Can you work these out from the model? Positions are in its coordinate system, mm. Face numbers are marked on the shaded views. Give positions to 0.01 mm unless a question says otherwise; leave off trailing zeros. Return JSON: item names as keys, results as strings. Group by question number.
Q1. Suppose I cut it at A-A, the plane y = -104.5. Count the separate pieces of the cut face and the enclosed holes in it, and give its area (3 significant figures).
Q2. I need wall thicknesses on line 1 along Z through (x, y) = (0, -60); line 2 along Y through (x, z) = (70, 57). Which ranges of each line are inside material? Lowest first, please. Write a range as [from, to].
Q3. Will these pins go through, and if not, where does the flat tip stop? pin 1 (4 mm diameter, centred on y = -73, z = -92, fed in from -X); pin 2 (5.5 mm diameter, centred on y = -88, z = 89, fed in from -X); pin 3 (1.7 mm diameter, centred on x = 0, y = -80.5, fed in from -Z); pin 4 (4 mm diameter, centred on y = -79.5, z = -0.5, fed in from +X).
Q4. Thinking about a two-plate mould opening in Z: for the marked faces 1, 2 and 3, which applies, pulls with the +Z half, pulls with the -Z half, needs draft (parallel to the pull), parting line crosses it, or undercut?
```python
from build123d import *

# Parameters (mm, degrees)
SKETCH1_R           = 94.2975
SKETCH1_R_2         = 89.662
BOSS_EXTRUDE1_DEPTH = 127
SKETCH5_W           = 3.429
SKETCH5_H           = 5.08
SKETCH5_W_2         = 5.08
SKETCH5_H_2         = 3.429
CUT_EXTRUDE1_DEPTH  = 127
CUT_EXTRUDE2_START  = -12.7
CUT_EXTRUDE2_DEPTH  = 107.95
CIRPATTERN1_COUNT   = 4
FILLET1_R           = 2.54


with BuildPart() as part:
    # Sketch1 → Boss-Extrude1 (new body)
    with BuildSketch(Plane(origin=(0, 0, 0), x_dir=(1, 0, 0), z_dir=(0, 1, 0))):
        Circle(SKETCH1_R)
        Circle(SKETCH1_R_2, mode=Mode.SUBTRACT)
    extrude(amount=-BOSS_EXTRUDE1_DEPTH)

    # Sketch5 → Cut-Extrude1 (cut)
    with BuildSketch(Plane(origin=(0, 0, 0), x_dir=(1, 0, 0), z_dir=(0, 1, 0))):
        with Locations((0, 93.360875)):
            Rectangle(SKETCH5_W, SKETCH5_H)
        with Locations((0, -93.360875)):
            Rectangle(SKETCH5_W, SKETCH5_H)
        with Locations((-93.360875, -0.0635)):
            Rectangle(SKETCH5_W_2, SKETCH5_H_2)
        with Locations((93.360875, -0.0635)):
            Rectangle(SKETCH5_W_2, SKETCH5_H_2)
    extrude(amount=-CUT_EXTRUDE1_DEPTH, mode=Mode.SUBTRACT)

    # Sketch7 → Cut-Extrude2 (cut)
    with BuildSketch(Plane(origin=(0, 0, 0), x_dir=(1, 0, 0), z_dir=(0, 1, 0)).offset(CUT_EXTRUDE2_START)):
        with BuildLine():
            Line((85.443727447, -27.178), (90.296039903, -27.178))
            ThreePointArc((90.296039903, -27.178), (66.654954519, -66.701840637), (27.1145, -90.315128279))
            Line((27.1145, -90.315128279), (27.1145, -85.463899594))
            ThreePointArc((27.1145, -85.463899594), (63.377047615, -63.424160063), (85.443727447, -27.178))
        make_face()
    cut_extrude2 = extrude(amount=-CUT_EXTRUDE2_DEPTH, mode=Mode.SUBTRACT)

    # CirPattern1: Cut-Extrude2 ×4 about axis
    cirpattern1_axis = Axis((0, 0, 0), (0, 1, 0))
    for i in range(1, CIRPATTERN1_COUNT):
        add(cut_extrude2.rotate(cirpattern1_axis, i * 360 / CIRPATTERN1_COUNT), mode=Mode.SUBTRACT)

    # Fillet1
    fillet1_edges = [part.edges().sort_by_distance(p)[0] for p in [
        (66.700852134, -127, -66.655943702),
        (-66.700852134, -127, -66.655943702),
        (-66.655943427, -127, 66.700852409),
        (66.655943427, -127, 66.700852409),
    ]]
    fillet(fillet1_edges, radius=FILLET1_R)


solid = part.part
```
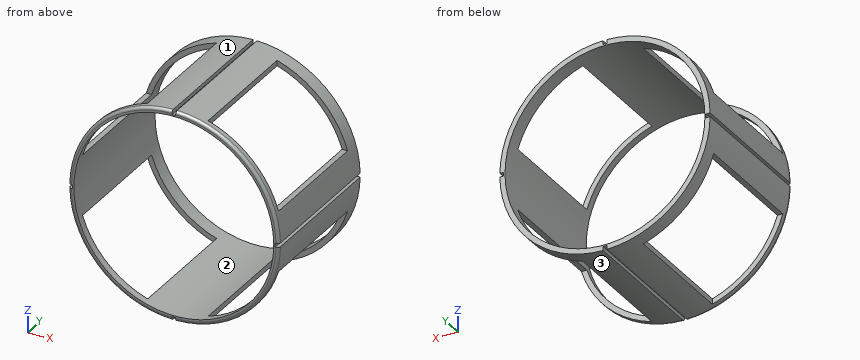
Ans:
{
 "1": {"separate pieces": "4", "enclosed holes": "0", "area": "974 mm^2"},
 "2": {"line 1": "z = [-90.82, -89.66], [89.66, 90.82]", "line 2": "y = [-127, -120.65], [-12.7, 0]"},
 "3": {"pin 1": "stops at x = -27.11", "pin 2": "stops at x = -27.18", "pin 3": "stops at z = -90.82", "pin 4": "stops at x = 94.28"},
 "4": {"face 1": "pulls with the +Z half", "face 2": "undercut", "face 3": "pulls with the -Z half"}
}
